```python
from build123d import *

# Parameters (mm, degrees)
BOSS_EXTRUDE1_DEPTH = 2.5
BOSS_EXTRUDE2_DEPTH = 8
FILLET2_R           = 1
CUT_EXTRUDE1_DEPTH  = 8
SKETCH4_R           = 2.3
CUT_EXTRUDE2_DEPTH  = 1.7
SKETCH5_R           = 1.15
CUT_EXTRUDE3_DEPTH  = 26.137422433
FILLET3_R           = 1


with BuildPart() as part:
    # Sketch1 → Boss-Extrude1 (new body)
    with BuildSketch(Plane.XY):
        with BuildLine():
            Line((15, -10), (-9.633249581, -10))
            ThreePointArc((-9.633249581, -10), (-15, 0), (-9.633249581, 10))
            Line((-9.633249581, 10), (15, 10))
            Line((15, 10), (15, -10))
        make_face()
    extrude(amount=BOSS_EXTRUDE1_DEPTH)

    # Sketch2 → Boss-Extrude2 (add)
    with BuildSketch(Plane(origin=(15, 0, 0), x_dir=(0, 0, -1), z_dir=(1, 0, 0))):
        with BuildLine():
            Line((0, -8.449489743), (0, -3.550510257))
            ThreePointArc((0, -3.550510257), (-1.5, -6), (0, -8.449489743))
        make_face()
        with BuildLine():
            Line((0, 3.550510257), (0, 8.449489743))
            ThreePointArc((0, 8.449489743), (-1.5, 6), (0, 3.550510257))
        make_face()
    extrude(amount=BOSS_EXTRUDE2_DEPTH)

    # Fillet2
    fillet2_edges = [part.edges().sort_by_distance(p)[0] for p in [
        (15, -6, 1.5),
        (15, 6, 1.5),
    ]]
    fillet(fillet2_edges, radius=FILLET2_R - 0.0001)  # a hair under: the kernel refuses the full size

    # Sketch3 → Cut-Extrude1 (cut)
    with BuildSketch(Plane(origin=(0, 0, 0), x_dir=(-1, 0, 0), z_dir=(0, 0, -1))):
        with BuildLine():
            Line((8, -4.8), (-3, -4.8))
            ThreePointArc((-3, -4.8), (-7.8, 0), (-3, 4.8))
            Line((-3, 4.8), (8, 4.8))
            ThreePointArc((8, 4.8), (12.8, 0), (8, -4.8))
        make_face()
    extrude(amount=-CUT_EXTRUDE1_DEPTH, mode=Mode.SUBTRACT)

    # Sketch4 → Cut-Extrude2 (cut)
    with BuildSketch(Plane.XY.offset(2.5)):
        with Locations((-5, 7.5)):
            Circle(SKETCH4_R)
        with Locations((11, 6)):
            Circle(SKETCH4_R)
        with Locations((11, -6)):
            Circle(SKETCH4_R)
        with Locations((-5, -7.5)):
            Circle(SKETCH4_R)
    extrude(amount=-CUT_EXTRUDE2_DEPTH, mode=Mode.SUBTRACT)

    # Sketch5 → Cut-Extrude3 (cut, through all)
    with BuildSketch(Plane.XY.offset(0.8)):
        with Locations((-5, 7.5)):
            Circle(SKETCH5_R)
        with Locations((11, 6)):
            Circle(SKETCH5_R)
        with Locations((11, -6)):
            Circle(SKETCH5_R)
        with Locations((-5, -7.5)):
            Circle(SKETCH5_R)
    extrude(amount=-CUT_EXTRUDE3_DEPTH, mode=Mode.SUBTRACT)

    # Fillet3
    fillet3_edges = [part.edges().sort_by_distance(p)[0] for p in [
        (-15, 0, 2.5),
    ]]
    fillet(fillet3_edges, radius=FILLET3_R)


solid = part.part
```
The listing builds one solid part. Answer for the finished solid, in the listing's coordinates (mm). A direction names the side the tool comes from. Coordinates: 2 decimals unless noted, no trailing zeros. Loops run counter-clockwise (first coordinate to the right, second up) from the corner with the lowest first, then second, coordinate; pieces in that order, holes last. Notation, with made-up numbers: (-1, 33.25) -> (52, 33.25) arc R9 ccw to (52, 45.25) -> close; hole circle Ø8 at (-10.5, 22.25). An arc over 180 degrees is marked (long way). Return JSON: item names as keys, results as strings. Group by question number.
(1) A cutting plane is placed at D-D on z = 2. Count the separate pieces of the cut face and the enclosed holes in it, and give its area (3 significant figures).
(2) A cutting plane is placed at A-A on y = 0. Write down the section's boundary in (x, z).
(3) Determine the mould class of faces 4 (the flat face through (23, -6, 1)), 5 (the flat face through (10, -5, 0.8)), 6 (the flat face through (3, -10, 1)), 7 (the cylindrical face through (-15, 0, 1)) for opening direction Y: released by +Y, released by -Y, zero draft, split by the parting line, or undercut.
(4) Find the intervals of material crossed by probe 1 along Y at (x, z) = (-5, 0.6); probe 2 along Y at (x, z) = (-5, 1.5); probe 3 along Y at (x, z) = (11, 1.95), in increasing order. Write a range as from..to.
(5) A cutting plane is placed at C-C on x = -1. Write down the section's boundary in (y, z).
(6) Given pin 1 Ø3.5 at (x, y) = (-4.5, 7.5) entering from +Z; pin 2 Ø7.5 at (x, y) = (11, -6) entering from +Z; pin 3 Ø1.5 at (x, y) = (-1.5, -3.5) entering from +Z; pin 4 Ø1 at (y, z) = (-3.5, 2) entering from +X, each flat-ended and moving along its own axis, determine where each tip first touches the part or whether it passes through.
(7) A cutting plane is placed at B-B on x = -5. Write down the section's boundary in (y, z), and give its area (3 significant figures).
(8) Which of the six approach directions +Z, -Z, +X, -X, +Y, -Y give full straight-line access (tool end or side, diameter ignored) to faces 1 (the cylindrical face through (-12.8, 0.1, 1.2)), 2 (the cylindrical face through (19.5, 6, 1.5)), 3 (the flat face through (10, 7, 0.8))?
The answers:
{
 "1": {"separate pieces": "1", "enclosed holes": "5", "area": "321 mm^2"},
 "2": {"outline": "(-15, 0) -> (-12.8, 0) -> (-12.8, 2.5) -> (-14, 2.5) arc R1 ccw to (-15, 1.5) -> close; (7.8, 0) -> (15, 0) -> (15, 2.5) -> (7.8, 2.5) -> close"},
 "3": {"face 4": "zero draft", "face 5": "undercut", "face 6": "released by -Y", "face 7": "split by the parting line"},
 "4": {"probe 1": "y = -10..-8.65, -6.35..-4.8, 4.8..6.35, 8.65..10", "probe 2": "y = -10..-9.8, -5.2..-4.8, 4.8..5.2, 9.8..10", "probe 3": "y = -10..-8.3, -3.7..3.7, 8.3..10"},
 "5": {"outline": "(-10, 0) -> (-4.8, 0) -> (-4.8, 2.5) -> (-10, 2.5) -> close; (4.8, 0) -> (10, 0) -> (10, 2.5) -> (4.8, 2.5) -> close"},
 "6": {"pin 1": "stops at z = 0.8", "pin 2": "stops at z = 2.5", "pin 3": "passes through", "pin 4": "stops at x = 15.01"},
 "7": {"outline": "(-10, 0) -> (-8.65, 0) -> (-8.65, 0.8) -> (-9.8, 0.8) -> (-9.8, 2.5) -> (-10, 2.5) -> close; (-6.35, 0) -> (-4.8, 0) -> (-4.8, 2.5) -> (-5.2, 2.5) -> (-5.2, 0.8) -> (-6.35, 0.8) -> close; (4.8, 0) -> (6.35, 0) -> (6.35, 0.8) -> (5.2, 0.8) -> (5.2, 2.5) -> (4.8, 2.5) -> close; (8.65, 0) -> (10, 0) -> (10, 2.5) -> (9.8, 2.5) -> (9.8, 0.8) -> (8.65, 0.8) -> close", "area": "6.68 mm^2"},
 "8": {"face 1": "+Z, -Z", "face 2": "+Z, +X", "face 3": "+Z"}
}
